Design review of the part built by this model. Coordinates are the model's own, in mm. A direction names the side the tool comes from. Round coordinates to 2 decimals unless told otherwise and drop trailing zeros. Loops run counter-clockwise (first coordinate to the right, second up) from the corner with the lowest first, then second, coordinate; pieces in that order, holes last. Notation, with made-up numbers: (25, -12) - (60, -12) arc R24 cw to (60, 6) - close; hole circle Ø8 at (-25.75, -25). An arc over 180 degrees is marked (long way). Use one line per item in the form item = value. Start each with the question number.
(1) We need section C-C, the plane y = 570. Write out the cut boundary in (x, z).
(2) The part is to be moulded in two halves that separate along X. For faces 4 (the flat face through (-180.2, 574, 10)), 5 (the flat face through (-159.04, 577, 2)), 6 (the flat face through (-142, 617, 10)), say which applies: released by +X, released by -X, zero draft, split by the parting line, or undercut.
(3) We need section D-D, the plane z = 8.75. Give the number of separate pieces and of enclosed holes in the cut face, then the cut area to 3 significant figures.
(4) We need section A-A, the plane y = 545. Write out the cut boundary in (x, z), then the cut area to 3 significant figures.
(5) We need section B-B, the plane x = -110. Write out the cut boundary in (y, z).
(6) Wall thickness on probe 1 along Y at (x, z) = (-118.5, 16.5); probe 2 along Y at (x, z) = (-140, 4.5); probe 3 along X at (y, z) = (530, 12.75): over which ranges is each line inside the solid? List them lowest first. Write a range as [from, to].
(7) For pin 1 (1 mm diameter, centred on x = -139, z = 5, fed in from -Y); pin 2 (2.5 mm diameter, centred on x = -117.5, y = 575.5, fed in from -Z); pin 3 (2 mm diameter, centred on y = 529.5, z = 17, fed in from -X), all flat-tipped, find the tip position at first contact; note any pin that passes through.
(8) Machinability: for faces 1 (the flat face through (-114.99, 591.59, 1.97)), 2 (the flat face through (-141.599, 521.835, 9.633)), 3 (the flat face through (-113, 470, 10)), which of the approach directions +Z, -Z, +X, -X, +Y, -Y give a long, thin tool a straight path to every point of the face, cutting with its end or side? Answer none if there is none.
from build123d import *

# Parameters (mm, degrees)
BOSS_EXTRUDE1_DEPTH  = 19
FILLET1_R            = 10
M5_CLEARANCE_HOLE2_D = 5.5
M5_CLEARANCE_HOLE1_D = 5.5
FILLET2_R            = 4
BOSS_EXTRUDE2_DEPTH  = 19
M8_CLEARANCE_HOLE1_D = 9
CUT_EXTRUDE2_DEPTH   = 4
SKETCH16_R           = 10
CUT_EXTRUDE3_DEPTH   = 5
CUT_EXTRUDE4_DEPTH   = 20
SKETCH19_R           = 10
CUT_EXTRUDE5_DEPTH   = 20


with BuildPart() as part:
    # Sketch1 → Boss-Extrude1 (new body)
    with BuildSketch(Plane.XY):
        with BuildLine():
            Line((-170.200000001, 540.824594888), (-129.309401077, 470))
            Line((-129.309401077, 470), (-93, 470))
            ThreePointArc((-93, 470), (-90.878679656, 470.878679656), (-90, 473))
            Line((-90, 473), (-90, 564.25527297))
            Line((-90, 564.25527297), (-116.225329238, 607))
            Line((-116.225329238, 607), (-170.200000001, 607))
            Line((-170.200000001, 607), (-170.200000001, 540.824594888))
        make_face()
    extrude(amount=BOSS_EXTRUDE1_DEPTH)

    # Fillet1
    fillet1_edges = [part.edges().sort_by_distance(p)[0] for p in [
        (-90, 564.25527297, 9.5),
        (-129.309401077, 470, 9.5),
        (-170.200000001, 540.824594888, 9.5),
    ]]
    fillet(fillet1_edges, radius=FILLET1_R)

    # M5 Clearance Hole2 (through all)
    with Locations(Plane(origin=(0, 0, 0), x_dir=(-1, 0, 0), z_dir=(0, 0, -1))):
        with Locations((117.000000001, 595), (117.000000001, 577), (163.000000001, 577), (163.000000001, 595)):
            Hole(M5_CLEARANCE_HOLE2_D / 2)

    # M5 Clearance Hole1 (through all)
    with Locations(Plane.XY.offset(19)):
        with Locations((-95, 545), (-125, 545), (-125, 475), (-95, 475), (-110, 490), (-110, 530)):
            Hole(M5_CLEARANCE_HOLE1_D / 2)

    # Fillet2
    fillet2_edges = [part.edges().sort_by_distance(p)[0] for p in [
        (-116.225329238, 607, 9.5),
        (-170.200000001, 607, 9.5),
    ]]
    fillet(fillet2_edges, radius=FILLET2_R)

    # Sketch11 → Boss-Extrude2 (add)
    with BuildSketch(Plane.XY.offset(19)):
        with BuildLine():
            ThreePointArc((-143.743157806, 475), (-140.082903769, 471.339745962), (-135.082903769, 470))
            Line((-135.082903769, 470), (-123.535898385, 470))
            ThreePointArc((-123.535898385, 470), (-128.535898385, 471.339745962), (-132.196152423, 475))
            Line((-132.196152423, 475), (-168.860254039, 538.504086813))
            ThreePointArc((-168.860254039, 538.504086813), (-169.859258264, 540.915896362), (-170.200000001, 543.504086813))
            Line((-170.200000001, 543.504086813), (-170.200000001, 603))
            ThreePointArc((-170.200000001, 603), (-169.028427125, 605.828427125), (-166.200000001, 607))
            Line((-166.200000001, 607), (-118.464037729, 607))
            ThreePointArc((-118.464037729, 607), (-116.510482263, 606.490504411), (-115.054590744, 605.091810521))
            Line((-115.054590744, 605.091810521), (-91.476382537, 566.661632408))
            ThreePointArc((-91.476382537, 566.661632408), (-90.37617086, 564.149073659), (-90, 561.432106106))
            Line((-90, 561.432106106), (-90, 473))
            ThreePointArc((-90, 473), (-90.878679656, 470.878679656), (-93, 470))
            Line((-93, 470), (-90, 470))
            ThreePointArc((-90, 470), (-82.928932188, 472.928932188), (-80, 480))
            Line((-80, 480), (-80, 561.432106106))
            ThreePointArc((-80, 561.432106106), (-80.75234172, 566.866041212), (-82.952765074, 571.89115871))
            Line((-82.952765074, 571.89115871), (-106.530973281, 610.321336823))
            ThreePointArc((-106.530973281, 610.321336823), (-111.626593598, 615.216765438), (-118.464037729, 617))
            Line((-118.464037729, 617), (-166.200000001, 617))
            ThreePointArc((-166.200000001, 617), (-176.099494937, 612.899494937), (-180.200000001, 603))
            Line((-180.200000001, 603), (-180.200000001, 543.504086813))
            ThreePointArc((-180.200000001, 543.504086813), (-179.518516526, 538.327705911), (-177.520508076, 533.504086813))
            Line((-177.520508076, 533.504086813), (-143.743157806, 475))
        make_face()
    extrude(amount=-BOSS_EXTRUDE2_DEPTH)

    # M8 Clearance Hole1 (through all)
    with Locations(Plane.XY.offset(19)):
        with Locations((-110, 530), (-110, 490)):
            Hole(M8_CLEARANCE_HOLE1_D / 2)

    # Sketch15 → Cut-Extrude2 (cut)
    with BuildSketch(Plane.XY):
        Polygon((-166.960000001, 579.286307066), (-166.960000001, 574.713692934), (-163.000000001, 572.427385868), (-159.040000001, 574.713692934), (-159.040000001, 579.286307066), (-163.000000001, 581.572614132), align=None)
        Polygon((-120.960000001, 579.286307066), (-120.960000001, 574.713692934), (-117.000000001, 572.427385868), (-113.040000001, 574.713692934), (-113.040000001, 579.286307066), (-117.000000001, 581.572614132), align=None)
        Polygon((-113.040000001, 592.713692934), (-117.000000001, 590.427385868), (-120.960000001, 592.713692934), (-120.960000001, 597.286307066), (-117.000000001, 599.572614132), (-113.040000001, 597.286307066), align=None)
        Polygon((-163.000000001, 590.427385868), (-166.960000001, 592.713692934), (-166.960000001, 597.286307066), (-163.000000001, 599.572614132), (-159.040000001, 597.286307066), (-159.040000001, 592.713692934), align=None)
    extrude(amount=CUT_EXTRUDE2_DEPTH, mode=Mode.SUBTRACT)

    # Sketch16 → Cut-Extrude3 (cut)
    with BuildSketch(Plane(origin=(0, 0, 19), x_dir=(-1, 0, 0), z_dir=(0, 0, -1))):
        with Locations((140.000000001, 577)):
            Circle(SKETCH16_R)
    extrude(amount=CUT_EXTRUDE3_DEPTH, mode=Mode.SUBTRACT)

    # Sketch18 → Cut-Extrude4 (cut)
    with BuildSketch(Plane.XY.offset(19)):
        Polygon((-130, 540.1), (-133.716421356, 540.1), (-137.641421356, 536.175), (-139.608578644, 536.175), (-143.533578644, 540.1), (-148.25, 540.1), (-148.25, 519.9), (-143.533578644, 519.9), (-139.608578644, 523.825), (-137.641421356, 523.825), (-133.716421356, 519.9), (-130, 519.9), align=None)
    extrude(amount=-CUT_EXTRUDE4_DEPTH, mode=Mode.SUBTRACT)

    # Sketch19 → Cut-Extrude5 (cut)
    with BuildSketch(Plane.XY.offset(14)):
        with Locations((-140.000000001, 577)):
            Circle(SKETCH19_R)
    extrude(amount=-CUT_EXTRUDE5_DEPTH, mode=Mode.SUBTRACT)


solid = part.part
Data:
q1.outline = (-180.2, 0) - (-147.14, 0) - (-147.14, 19) - (-180.2, 19) - close; (-132.86, 0) - (-81.93, 0) - (-81.93, 19) - (-132.86, 19) - close
q2.face_4 = released by -X
q2.face_5 = undercut
q2.face_6 = zero draft
q3.separate_pieces = 1
q3.enclosed_holes = 12
q3.area = 11,600 mm^2
q4.outline = (-180.2, 0) - (-127.75, 0) - (-127.75, 19) - (-180.2, 19) - close; (-122.25, 0) - (-97.75, 0) - (-97.75, 19) - (-122.25, 19) - close; (-92.25, 0) - (-80, 0) - (-80, 19) - (-92.25, 19) - close
q4.area = 1,690 mm^2
q5.outline = (470, 0) - (485.5, 0) - (485.5, 19) - (470, 19) - close; (494.5, 0) - (525.5, 0) - (525.5, 19) - (494.5, 19) - close; (534.5, 0) - (614.15, 0) - (614.15, 19) - (534.5, 19) - close
q6.probe_1 = [470, 574.7], [579.3, 592.7], [597.3, 617]
q6.probe_2 = [471.29, 523.43], [536.57, 567], [587, 617]
q6.probe_3 = [-175.5, -148.25], [-130, -114.5], [-105.5, -80]
q7.pin_1 = 470.6
q7.pin_2 = 4
q7.pin_3 = -175.79
q8.face_1 = -Z
q8.face_2 = +Z, -Z
q8.face_3 = +Z, -Z, +X, -X, -Y
